For this review, take the finished solid that the model builds, in its own axes (mm). Face numbers are marked on the shaded views. A direction names the side the tool comes from. Coordinates: 2 decimals unless noted, no trailing zeros. Order: outer loops, then holes, each group sorted by start corner. A loop starts at its lowest first (then second) coordinate and runs counter-clockwise, first axis right, second up. Notation, with made-up numbers: (82.25, 22) -> (97.25, 22) arc R11 ccw to (97.25, 36) -> close; hole circle Ø11 at (-19.5, -13). An arc over 180 degrees is marked (long way). Write item = value, one per line. Start each with the question number.
1) Consider section B-B on y = 0. Give the boundary of the cut face in (x, z).
2) Wall thickness on probe 1 along Y at (x, z) = (40.55, -36); probe 2 along Y at (x, z) = (39.3, -36); probe 3 along Z at (x, y) = (10, -2.75): over which ranges is each line inside the solid? List them lowest first. Write a range as [from, to].
3) Consider section A-A on x = 7. Give the boundary of the cut face in (y, z).
4) Draft analysis for pull direction Y (two halves, no side actions). For the marked faces 1 and 2, state which applies: +Y half, -Y half, draft (parallel to the pull), parting line (faces both ways), or undercut.
5) Consider section C-C on z = 0. Give the boundary of the cut face in (x, y), and give its area (3 significant figures).
6) Machinability: for the marked faces 3, 4, 5 and 6, which of the approach directions +Z, -Z, +X, -X, +Y, -Y give a long, thin tool a straight path to every point of the face, cutting with its end or side? Answer none if there is none.
7) Insertion check: pin 1 Ø9.5 at (y, z) = (-4, 37) entering from -X; pin 2 Ø10 at (x, y) = (34, -8) entering from +Z; pin 3 Ø9 at (x, y) = (27, -0.5) entering from +Z. Each pin has a flat end and moves straight along its axis. Give the tip position at first contact, or say it passes through.
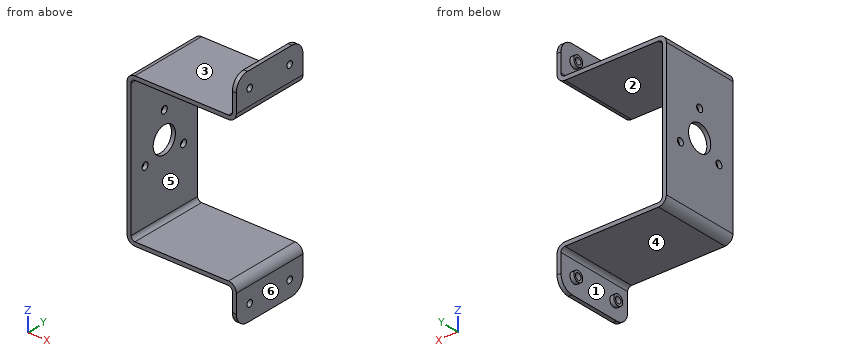
Autodesk Inventor part; units mm, degrees
ref_plane "YZ Plane" through (0, 0, 0) normal (1, 0, 0) x (0, 1, 0)
ref_plane "XZ Plane" through (0, 0, 0) normal (0, 1, 0) x (-1, 0, 0)
ref_plane "XY Plane" through (0, 0, 0) normal (0, 0, 1) x (1, 0, 0)
sketch "スケッチ1" plane through (0, 0, 0) normal (1, 0, 0) x (0, 1, 0)
  line L0 (-15, -27) -> (-15, 27)
  line L1 (-15, 27) -> (15, 27)
  line L2 (15, 27) -> (15, -27)
  line L3 (15, -27) -> (-15, -27)
  line L4 (-15, -27) -> (15, 27) construction
  line L5 (-15, 27) -> (15, -27) construction
  point P0 (0, 0)
  dimension "d0" = 30
  dimension "d1" = 54
extrude "プレート1" add sketch "スケッチ1" along normal blind 1.5
sketch "スケッチ2" plane through (1.5, -15, 27) normal (0, 0, 1) x (1, 0, 0)
  line L0 (0, 30) -> (0, 0)
  line L1 (0, 0) -> (38.5, 0)
  line L2 (38.5, 0) -> (38.5, 30)
  line L3 (38.5, 30) -> (0, 30)
edge flange "フランジ1" height 40 angle 90 thickness 1.5 bend radius 1.5 thickness toward (0, 0, 1) relief tear relief width 1.5 relief depth 0.75 corner gap 1.5 corner form 0 edges at (1.5, 0, 27) (1.5, 0, -27) wall of the first edge with corners at (1.5, 15, 27) (1.5, -15, 27) (40, -15, 27) (40, 15, 27)
bend "曲げ1"
corner "コーナー1"
sketch "スケッチ3" plane through (40, 15, 28.5) normal (1, 0, 0) x (0, 1, 0)
  line L0 (-30, 0) -> (0, 0)
  line L1 (0, 0) -> (0, 13.5)
  line L2 (0, 13.5) -> (-30, 13.5)
  line L3 (-30, 13.5) -> (-30, 0)
edge flange "フランジ2" height 15 angle 90 thickness 1.5 bend radius 1.5 thickness toward (1, 0, 0) relief tear relief width 1.5 relief depth 0.75 corner gap 1.5 corner form 0 edges at (40, 0, 28.5) (40, 0, -28.5) wall of the first edge with corners at (40, -15, 28.5) (40, 15, 28.5) (40, 15, 42) (40, -15, 42)
bend "曲げ2"
corner "コーナー2"
sketch "スケッチ4" plane through (0, 0, 0) normal (-1, 0, 0) x (0, 0, 1)
  circle A0 centre (0, 0) radius 5
  circle A1 centre (10, 0) radius 1.35
  circle A2 centre (-5, 8.6603) radius 1.35
  circle A3 centre (-5, -8.6603) radius 1.35
  dimension "d23" = 10
  dimension "d24" = 2.7
  dimension "d25" = 0
  dimension "d26" = 10
  dimension "d29" = 360
extrude "押し出し1" cut sketch "スケッチ4" against normal blind 2
sketch "スケッチ6" plane through (40, -15, 42) normal (-1, 0, 0) x (0, 0, 1)
  circle A0 centre (-6, 24) radius 2
  line L0 (-12, 30) -> (0, 30)
  line L1 (0, 0) -> (0, 30)
  circle A1 centre (-6, 6) radius 2
  circle A2 centre (-78, 24) radius 2
  circle A3 centre (-78, 6) radius 2
  point P0 (-42, 15)
  dimension "d41" = 4
  dimension "d42" = 4
  dimension "d43" = 4
  dimension "d46" = 18
  dimension "d49" = 72
extrude "押し出し3" add sketch "スケッチ6" along normal blind 1.5
sketch "スケッチ7" plane through (38.5, 9, 36) normal (-1, 0, 0) x (0, 0, 1)
  circle A0 centre (0, 0) radius 2
  circle A1 centre (0, -18) radius 2
  circle A2 centre (-72, -18) radius 2
  circle A3 centre (-72, 0) radius 2
  circle A4 centre (0, 0) radius 2
  circle A5 centre (0, -18) radius 2
  circle A6 centre (-72, -18) radius 2
  point P0 (-36, -9)
hole "穴1" at (38.5, 9, 36) at (38.5, -9, 36) at (38.5, 9, -36) at (38.5, -9, -36) direction (1, 0, 0) diameter 2.459 depth 3
fillet "フィレット1" radius 5 4 edges at (40.75, 15, 42) (40.75, -15, 42) (40.75, 15, -42) (40.75, -15, -42)
equation "\"d59\" = Thickness"
equation "\"BendRadius\" = Thickness"
equation "\"BendReliefWidth\" = Thickness"
equation "\"BendReliefDepth\" = 0.5 * Thickness"
equation "\"CornerReliefSize\" = 4 * Thickness"
equation "\"MinimumRemnant\" = 2 * Thickness"
equation "\"TransitionRadius\" = BendRadius"
equation "\"JacobiRadiusSize\" = BendRadius"
equation "\"GapSize\" = Thickness"
properties part number "hand_box2" material "アルミニウム 5052"
Answer sheet:
q1.outline = (0, -25.5) arc R3 ccw to (3, -28.5) -> (38.5, -28.5) arc R1.5 cw to (40, -30) -> (40, -42) -> (41.5, -42) -> (41.5, -30) arc R3 ccw to (38.5, -27) -> (3, -27) arc R1.5 cw to (1.5, -25.5) -> (1.5, -5) -> (0, -5) -> close; (0, 5) -> (1.5, 5) -> (1.5, 8.65) -> (0, 8.65) -> close; (0, 11.35) -> (1.5, 11.35) -> (1.5, 25.5) arc R1.5 cw to (3, 27) -> (38.5, 27) arc R3 ccw to (41.5, 30) -> (41.5, 42) -> (40, 42) -> (40, 30) arc R1.5 cw to (38.5, 28.5) -> (3, 28.5) arc R3 ccw to (0, 25.5) -> close
q2.probe_1 = [-15, -10.23], [-7.77, 7.77], [10.23, 15]
q2.probe_2 = [-11, -10.23], [-7.77, -7], [7, 7.77], [10.23, 11]
q2.probe_3 = [-28.5, -27], [27, 28.5]
q3.outline = (-15, -28.5) -> (15, -28.5) -> (15, -27) -> (-15, -27) -> close; (-15, 27) -> (15, 27) -> (15, 28.5) -> (-15, 28.5) -> close
q4.face_1 = undercut
q4.face_2 = draft
q5.outline = (0, -15) -> (1.5, -15) -> (1.5, -5) -> (0, -5) -> close; (0, 5) -> (1.5, 5) -> (1.5, 15) -> (0, 15) -> close
q5.area = 30.0 mm2
q6.face_3 = +Z, -X, +Y, -Y
q6.face_4 = -Z, -X, +Y, -Y
q6.face_5 = +X, +Y, -Y
q6.face_6 = +Z, -Z, +X, +Y, -Y
q7.pin_1 = 38.5
q7.pin_2 = 38
q7.pin_3 = 28.5
